The model under review builds one solid part; all positions refer to its coordinate system, in mm. A direction names the side the tool comes from. Round coordinates to 2 decimals unless told otherwise and drop trailing zeros. Write each loop counter-clockwise with the first axis right and the second up, starting at its lowest first coordinate (ties: lowest second). Pieces come first, ordered by that corner, then holes. Notation, with made-up numbers: (30.25, 65) - (77.25, 65) arc R13 ccw to (77.25, 76) - close; hole circle Ø2 at (83.5, 28). An arc over 180 degrees is marked (long way). Write each question's results on one line, items separated by ' | '.
```python
from build123d import *

# Parameters (mm, degrees)
BOSS_EXTRUDE5_DEPTH = 80
BOSS_EXTRUDE6_DEPTH = 20
SKETCH6_W           = 10
SKETCH6_H           = 50
CUT_EXTRUDE5_DEPTH  = 222
SKETCH7_W           = 30
SKETCH7_H           = 15
CUT_EXTRUDE6_DEPTH  = 222
CUT_EXTRUDE7_DEPTH  = 10
CUT_EXTRUDE8_DEPTH  = 10
BOSS_EXTRUDE9_DEPTH = 10
CUT_EXTRUDE14_DEPTH = 30


with BuildPart() as part:
    # Sketch1 → Boss-Extrude5 (new body)
    with BuildSketch(Plane.XY):
        with BuildLine():
            Line((80, -80), (80, -30))
            ThreePointArc((80, -30), (65, -8.333333333), (40, 0))
            ThreePointArc((40, 0), (0, -40), (-40, 0))
            Line((-40, 0), (-80, 0))
            ThreePointArc((-80, 0), (-56.568542495, -56.568542495), (0, -80))
            Line((0, -80), (80, -80))
        make_face()
    extrude(amount=BOSS_EXTRUDE5_DEPTH)

    # Sketch4 → Boss-Extrude6 (add)
    with BuildSketch(Plane(origin=(0, 0, 0), x_dir=(-1, 0, 0), z_dir=(0, 0, -1))):
        with BuildLine():
            Line((20, 0), (40, 0))
            ThreePointArc((40, 0), (0, -40), (-40, 0))
            Line((-40, 0), (-20, 0))
            ThreePointArc((-20, 0), (0, -20), (20, 0))
        make_face()
    extrude(amount=-BOSS_EXTRUDE6_DEPTH)

    # Sketch6 → Cut-Extrude5 (cut)
    with BuildSketch(Plane(origin=(-80, 0, 0), x_dir=(0, 0, -1), z_dir=(1, 0, 0))):
        with Locations((-75, -25)):
            Rectangle(SKETCH6_W, SKETCH6_H)
    extrude(amount=CUT_EXTRUDE5_DEPTH, mode=Mode.SUBTRACT)

    # Sketch7 → Cut-Extrude6 (cut)
    with BuildSketch(Plane(origin=(-80, 0, 0), x_dir=(0, 0, -1), z_dir=(1, 0, 0))):
        with Locations((-55, -7.5)):
            Rectangle(SKETCH7_W, SKETCH7_H)
    extrude(amount=CUT_EXTRUDE6_DEPTH, mode=Mode.SUBTRACT)

    # Sketch9 → Cut-Extrude7 (cut)
    with BuildSketch(Plane.XY.offset(70)):
        with BuildLine():
            Line((72.015621187, -15), (60, -15))
            Line((60, -15), (60, -50))
            Line((60, -50), (80, -50))
            Line((80, -50), (80, -30))
            ThreePointArc((80, -30), (76.780598469, -22.088651257), (72.015621187, -15))
        make_face()
    extrude(amount=-CUT_EXTRUDE7_DEPTH, mode=Mode.SUBTRACT)

    # Sketch10 → Cut-Extrude8 (cut)
    with BuildSketch(Plane.XY.offset(70)):
        with BuildLine():
            Line((60, -50), (60, -15))
            Line((60, -15), (47.080992435, -15))
            ThreePointArc((47.080992435, -15), (28.601457744, -40.330339745), (-1.224989992, -50))
            Line((-1.224989992, -50), (60, -50))
        make_face()
    extrude(amount=-CUT_EXTRUDE8_DEPTH, mode=Mode.SUBTRACT)

    # Sketch11 → Boss-Extrude9 (add)
    with BuildSketch(Plane.XY.offset(60)):
        with BuildLine():
            Line((60, -50), (80, -50))
            Line((80, -50), (80, -30))
            ThreePointArc((80, -30), (76.780598469, -22.088651257), (72.015621187, -15))
            Line((72.015621187, -15), (70, -15))
            Line((70, -15), (60, -15))
            Line((60, -15), (60, -50))
        make_face()
    extrude(amount=BOSS_EXTRUDE9_DEPTH)

    # Sketch15 → Cut-Extrude14 (cut)
    with BuildSketch(Plane.XY.offset(70)):
        with BuildLine():
            Line((47.080992435, -15), (37.080992435, -15))
            ThreePointArc((37.080992435, -15), (0, -40), (-37.080992435, -15))
            Line((-37.080992435, -15), (-78.581168228, -15))
            ThreePointArc((-78.581168228, -15), (-72.654636407, -33.485874761), (-62.449979984, -50))
            Line((-62.449979984, -50), (-1.224989992, -50))
            ThreePointArc((-1.224989992, -50), (28.601457744, -40.330339745), (47.080992435, -15))
        make_face()
    extrude(amount=-CUT_EXTRUDE14_DEPTH, mode=Mode.SUBTRACT)


solid = part.part
```
Q1. We need section D-D (x = 10.5). State the section outline as (y, z) points, plus the area to 3 significant figures.
Evaluation:
outline: (-80, 0) - (-17.02, 0) - (-17.02, 20) - (-38.6, 20) - (-38.6, 40) - (-48.63, 40) - (-48.63, 60) - (-50, 60) - (-50, 80) - (-80, 80) - close | area: 3,320 mm^2
Q2. We need section A-A (z = 22). State the section outline as (x, y) points, plus the area to 3 significant figures.
Evaluation:
outline: (-80, 0) arc R80 ccw to (0, -80) - (80, -80) - (80, -30) arc R41.67 ccw to (40, 0) arc R40 cw to (-40, 0) - close | area: 8,600 mm^2
Q3. We need section C-C (y = -43.5). State the section outline as (x, z) points, plus the area to 3 significant figures.
Evaluation:
outline: (-67.14, 0) - (80, 0) - (80, 70) - (60, 70) - (60, 60) - (23.65, 60) - (23.65, 40) - (-67.14, 40) - close | area: 7,210 mm^2
Q4. The part is to be moulded in two halves that separate along X. For faces 1 (the flat face through (-56, 0, 20)), 2 (the cylindrical face through (0.88, -39.99, 29.86)), 3 (the cylindrical face through (69.759, -12.503, 26.732)), 4 (the cylindrical face through (28.24, -40.59, 50.14)), say which applies: released by +X, released by -X, zero draft, split by the parting line, or undercut.
Evaluation:
face 1: zero draft | face 2: undercut | face 3: released by +X | face 4: released by -X
Q5. For probe 1 along Y at (x, z) = (48.5, 71); probe 2 along Z at (x, y) = (29, -41); probe 3 along Z at (x, y) = (-21, -40.5), list the stretches that pass through material, from the lowest coordinate up.
Evaluation:
probe 1: y = -80 to -50 | probe 2: z = 0 to 60 | probe 3: z = 0 to 40
Q6. Insertion check: P1, Ø20, axis at x = 22, z = 52, coming from the +Y side; P2, Ø17.5, axis at x = 41, y = -25, coming from the +Z side; P3, Ø11, axis at y = -25, z = 66.5, coming from the -X side. Each pin has a flat end and moves straight along its axis. Give the tip position at first contact, or say it passes through.
Evaluation:
P1: stops at y = -37.64 | P2: stops at z = 60 | P3: stops at x = 60
Q7. We need section B-B (x = 50). State the section outline as (y, z) points, plus the area to 3 significant figures.
Evaluation:
outline: (-80, 0) - (-1.22, 0) - (-1.22, 40) - (-15, 40) - (-15, 60) - (-50, 60) - (-50, 80) - (-80, 80) - close | area: 5,050 mm^2
Q8. Tool access review of faces 5 (the flat face through (-1, -24, 20)), 6 (the flat face through (70, -32, 70)), 7 (the flat face through (60, -32, 65)), 8 (the cylindrical face through (-46.604, -65.024, 30.551)), 9 (the flat face through (24, -65, 80)): name each direction out of +Z, -Z, +X, -X, +Y, -Y from which nothing blocks a thin tool from reaching the whole face with its end or side.
Evaluation:
face 5: +Z, +Y | face 6: +Z, +X, -X, +Y | face 7: +Z, -X, +Y | face 8: +Z, -Z, -X, -Y | face 9: +Z, +X, -X, +Y, -Y
